Build history of the part. All positions in model axes, mm. Face numbers are marked on the shaded views. A direction names the side the tool comes from. Round coordinates to 2 decimals unless told otherwise and drop trailing zeros. Order: outer loops, then holes, each group sorted by start corner. A loop starts at its lowest first (then second) coordinate and runs counter-clockwise, first axis right, second up. Notation, with made-up numbers: (17.25, 84.25) - (52.25, 84.25) arc R10 cw to (52.25, 97.25) - close; hole circle Ø4 at (86, 21). An arc over 180 degrees is marked (long way). One line per question, with ' | ' between items. Start each with the question number.
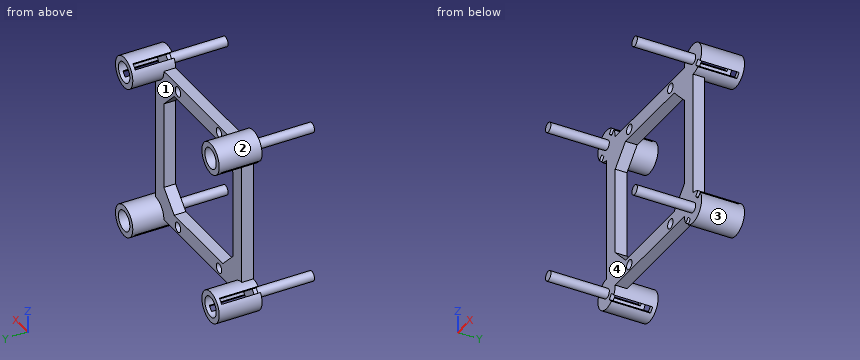
from build123d import *

# Parameters (mm, degrees)
BOSS_EXTRUDE1_DEPTH      = 6
SKETCH2_R                = 2.5
CUT_EXTRUDE1_DEPTH       = 69.14690015
BOSS_EXTRUDE2_DEPTH      = 16
BOSS_EXTRUDE2_DEPTH_BACK = 4
SKETCH4_R                = 8
CUT_EXTRUDE2_DEPTH       = 20
SKETCH7_R                = 5.25
CUT_EXTRUDE3_DEPTH       = 20
SKETCH8_R                = 2.5
BOSS_EXTRUDE3_DEPTH      = 30


with BuildPart() as part:
    # Sketch1 → Boss-Extrude1 (new body)
    with BuildSketch(Plane(origin=(0, 0, 0), x_dir=(1, 0, 0), z_dir=(0, 1, 0))):
        with BuildLine():
            Line((-32, -40), (32, -40))
            ThreePointArc((32, -40), (45.656854249, -45.656854249), (40, -32))
            Line((40, -32), (40, 32))
            ThreePointArc((40, 32), (45.656854249, 45.656854249), (32, 40))
            Line((32, 40), (-32, 40))
            ThreePointArc((-32, 40), (-45.656854249, 45.656854249), (-40, 32))
            Line((-40, 32), (-40, -32))
            ThreePointArc((-40, -32), (-45.656854249, -45.656854249), (-32, -40))
        make_face()
        Polygon((-22.5, 32), (22.5, 32), (32, 22.5), (32, -22.5), (22.5, -32), (-22.5, -32), (-32, -22.5), (-32, 22.5), align=None, mode=Mode.SUBTRACT)
    extrude(amount=BOSS_EXTRUDE1_DEPTH)

    # Sketch2 → Cut-Extrude1 (cut, through all)
    with BuildSketch(Plane.XZ):
        with Locations(Location((-19, -36.5, 0), (0, 0, 270))):
            Circle(SKETCH2_R)
        with Locations(Location((19, -36.5, 0), (0, 0, 270))):
            Circle(SKETCH2_R)
        with Locations(Location((19, 36.5, 0), (0, 0, 270))):
            Circle(SKETCH2_R)
        with Locations(Location((-19, 36.5, 0), (0, 0, 270))):
            Circle(SKETCH2_R)
    extrude(amount=-CUT_EXTRUDE1_DEPTH, mode=Mode.SUBTRACT)

    # Sketch4 → Boss-Extrude2 (add, two sides: drawn at the far end of the back side and taken through both)
    with BuildSketch(Plane(origin=(0, 6, 0), x_dir=(1, 0, 0), z_dir=(0, 1, 0)).offset(-BOSS_EXTRUDE2_DEPTH_BACK)):
        with Locations(Location((-40, 40, 0), (0, 0, 270))):
            Circle(SKETCH4_R)
        with Locations(Location((40, 40, 0), (0, 0, 270))):
            Circle(SKETCH4_R)
        with Locations(Location((40, -40, 0), (0, 0, 90))):
            Circle(SKETCH4_R)
        with Locations(Location((-40, -40, 0), (0, 0, 90))):
            Circle(SKETCH4_R)
    extrude(amount=BOSS_EXTRUDE2_DEPTH + BOSS_EXTRUDE2_DEPTH_BACK)

    # Sketch5 → Cut-Extrude2 (cut)
    with BuildSketch(Plane.XZ):
        with BuildLine():
            Line((-35.504132479, 46.617187865), (-37.525126266, 44.596194078))
            Line((-37.525126266, 44.596194078), (-35.403805922, 42.474873734))
            Line((-35.403805922, 42.474873734), (-33.382812135, 44.495867521))
            ThreePointArc((-33.382812135, 44.495867521), (-34.343145751, 45.656854249), (-35.504132479, 46.617187865))
        make_face()
        with BuildLine():
            Line((-44.596194078, 37.525126266), (-46.617187865, 35.504132479))
            ThreePointArc((-46.617187865, 35.504132479), (-45.656854249, 34.343145751), (-44.495867521, 33.382812135))
            Line((-44.495867521, 33.382812135), (-42.474873734, 35.403805922))
            Line((-42.474873734, 35.403805922), (-44.596194078, 37.525126266))
        make_face()
        with BuildLine():
            Line((35.403805922, 42.474873734), (37.525126266, 44.596194078))
            Line((37.525126266, 44.596194078), (35.504132479, 46.617187865))
            ThreePointArc((35.504132479, 46.617187865), (34.343145751, 45.656854249), (33.382812135, 44.495867521))
            Line((33.382812135, 44.495867521), (35.403805922, 42.474873734))
        make_face()
        with BuildLine():
            ThreePointArc((44.495867521, 33.382812135), (45.656854249, 34.343145751), (46.617187865, 35.504132479))
            Line((46.617187865, 35.504132479), (44.596194078, 37.525126266))
            Line((44.596194078, 37.525126266), (42.474873734, 35.403805922))
            Line((42.474873734, 35.403805922), (44.495867521, 33.382812135))
        make_face()
        with BuildLine():
            Line((44.596194078, -37.525126266), (46.617187865, -35.504132479))
            ThreePointArc((46.617187865, -35.504132479), (45.656854249, -34.343145751), (44.495867521, -33.382812135))
            Line((44.495867521, -33.382812135), (42.474873734, -35.403805922))
            Line((42.474873734, -35.403805922), (44.596194078, -37.525126266))
        make_face()
        with BuildLine():
            Line((35.504132479, -46.617187865), (37.525126266, -44.596194078))
            Line((37.525126266, -44.596194078), (35.403805922, -42.474873734))
            Line((35.403805922, -42.474873734), (33.382812135, -44.495867521))
            ThreePointArc((33.382812135, -44.495867521), (34.343145751, -45.656854249), (35.504132479, -46.617187865))
        make_face()
        with BuildLine():
            ThreePointArc((-44.495867521, -33.382812135), (-45.656854249, -34.343145751), (-46.617187865, -35.504132479))
            Line((-46.617187865, -35.504132479), (-44.596194078, -37.525126266))
            Line((-44.596194078, -37.525126266), (-42.474873734, -35.403805922))
            Line((-42.474873734, -35.403805922), (-44.495867521, -33.382812135))
        make_face()
        with BuildLine():
            Line((-35.403805922, -42.474873734), (-37.525126266, -44.596194078))
            Line((-37.525126266, -44.596194078), (-35.504132479, -46.617187865))
            ThreePointArc((-35.504132479, -46.617187865), (-34.343145751, -45.656854249), (-33.382812135, -44.495867521))
            Line((-33.382812135, -44.495867521), (-35.403805922, -42.474873734))
        make_face()
    extrude(amount=-CUT_EXTRUDE2_DEPTH, mode=Mode.SUBTRACT)

    # Sketch7 → Cut-Extrude3 (cut)
    with BuildSketch(Plane(origin=(0, 22, 0), x_dir=(1, 0, 0), z_dir=(0, 1, 0))):
        with Locations(Location((40, 40, 0), (0, 0, 270))):
            Circle(SKETCH7_R)
        with Locations(Location((40, -40, 0), (0, 0, 270))):
            Circle(SKETCH7_R)
        with Locations(Location((-40, -40, 0), (0, 0, 270))):
            Circle(SKETCH7_R)
        with Locations(Location((-40, 40, 0), (0, 0, 270))):
            Circle(SKETCH7_R)
    extrude(amount=-CUT_EXTRUDE3_DEPTH, mode=Mode.SUBTRACT)

    # Sketch8 → Boss-Extrude3 (add)
    with BuildSketch(Plane.XZ):
        with Locations(Location((-40, 40, 0), (0, 0, 90))):
            Circle(SKETCH8_R)
        with Locations(Location((40, 40, 0), (0, 0, 90))):
            Circle(SKETCH8_R)
        with Locations(Location((40, -40, 0), (0, 0, 90))):
            Circle(SKETCH8_R)
        with Locations(Location((-40, -40, 0), (0, 0, 90))):
            Circle(SKETCH8_R)
    extrude(amount=BOSS_EXTRUDE3_DEPTH)


solid = part.part
Item 1: Slice it at D-D (y = -15). Write the cut outline in (x, z).
Item 2: Wall check: line 1 along X through (y, z) = (8, 40); line 2 along X through (y, z) = (4, 36). Give the ranges that are in metal, low to high. Write a range as [from, to].
Item 3: Slice it at B-B (z = 2). Write the cut outline in (x, y).
Item 4: Pin check, flat tips, straight feed: pin 1 (6.5 mm diameter, centred on x = 0.5, y = 3.5, fed in from -Z); pin 2 (8 mm diameter, centred on x = 34, z = 6.5, fed in from +Y); pin 3 (6.5 mm diameter, centred on y = 3, z = -3.5, fed in from -X); pin 4 (3 mm diameter, centred on x = -19, z = 36.5, fed in from +Y). Stop position of each tip, or through.
Item 5: 3-axis set-ups, long thin cutter, end or side, ignore diameter. For the marked faces 3 and 4: which of +Z, -Z, +X, -X, +Y, -Y reach the whole face in a straight line?
Item 6: Slice it at A-A (x = -9). Write the cut outline in (y, z).
Item 7: Pull direction Z, two halves, no side cores. Call the marked faces 1 and 2: released by +Z, released by -Z, zero draft, split by the parting line, or undercut.
Item 8: Slice it at C-C (x = 19). Write the cut outline in (y, z).
A:
1) outline: circle Ø5 at (-40, -40); circle Ø5 at (-40, 40); circle Ø5 at (40, -40); circle Ø5 at (40, 40)
2) line 1: [-48, -45.25], [-34.75, -32], [32, 34.75], [45.25, 48] | line 2: [-46.93, -46.12], [-36.6, -21.45], [-16.55, 16.55], [21.45, 36.6], [46.12, 46.93]
3) outline: (-40, 0) - (-32, 0) - (-32, 6) - (-40, 6) - close; (32, 0) - (40, 0) - (40, 6) - (32, 6) - close
4) pin 1: z = -40 | pin 2: y = 6 | pin 3: x = -40 | pin 4: through
5) face 3: +Y | face 4: -Y
6) outline: (0, -40) - (6, -40) - (6, -32) - (0, -32) - close; (0, 32) - (6, 32) - (6, 40) - (0, 40) - close
7) face 1: undercut | face 2: undercut
8) outline: (0, -40) - (6, -40) - (6, -39) - (0, -39) - close; (0, -34) - (6, -34) - (6, -32) - (0, -32) - close; (0, 32) - (6, 32) - (6, 34) - (0, 34) - close; (0, 39) - (6, 39) - (6, 40) - (0, 40) - close
